For this review, take the finished solid that the model builds, in its own axes (mm). Face numbers are marked on the shaded views. A direction names the side the tool comes from. Give positions to 0.01 mm unless a question says otherwise; leave off trailing zeros. Write each loop counter-clockwise with the first axis right and the second up, starting at its lowest first coordinate (ties: lowest second). Pieces come first, ordered by that corner, then holes.
Q1. Mouldability with a two-part tool opening along Z and no side actions: class the marked faces 1, 2 and 3 as released by +Z, released by -Z, zero draft, split by the parting line, or undercut.
Q2. For line 1 (Z direction, x = 8.5, y = -12); line 2 (Y direction, x = 12.5, z = 1.25); line 3 (Y direction, x = 9.25, z = 7.5), list the stretches that pass through material, from the lowest coordinate up.
Q3. Machinability: for the marked faces 4, 5, 6, 7 and 8, which of the approach directions +Z, -Z, +X, -X, +Y, -Y give a long, thin tool a straight path to every point of the face, cutting with its end or side? Answer none if there is none.
Q4. We need section C-C (x = 13.75). Write out the cut boundary in (y, z).
Q5. We need section A-A (y = -14.25). Write out the cut boundary in (x, z).
Q6. Insertion check: P1, Ø6, axis at x = -6.5, y = -12.5, coming from the +Z side; P2, Ø8, axis at x = -4.5, y = -16.5, coming from the +Z side; P3, Ø1.5, axis at y = -3.5, z = 1.5, coming from the -X side. Each pin has a flat end and moves straight along its axis. Give the tip position at first contact, or say it passes through.
Q7. We need section B-B (x = 1.75). Write out the cut boundary in (y, z).
Q8. We need section D-D (z = 1.75). Write out the cut boundary in (x, y), then the cut area to 3 significant figures.
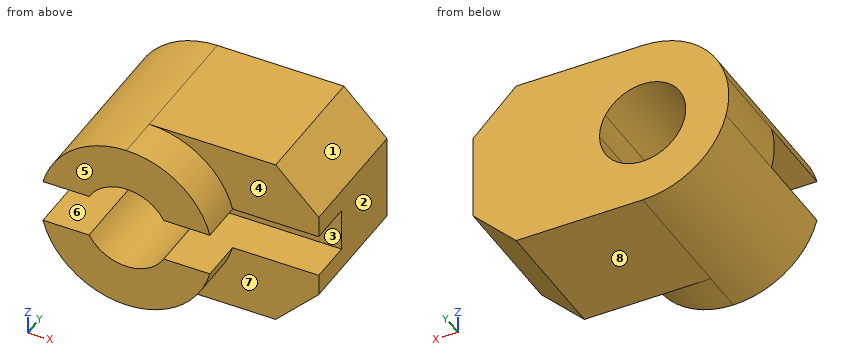
```python
from build123d import *

# Parameters (mm, degrees)
F1_DEPTH = 20
F2_DEPTH = 15
F3_DEPTH = 10


with BuildPart() as f1:
    # F0 (on Front) → F1 (new body)
    with BuildSketch(Plane.XZ):
        with BuildLine():
            ThreePointArc((-4.3301270189, 2.5), (0, 5), (4.3301270189, 2.5))
            Line((4.3301270189, 2.5), (9.6824583655, 2.5))
            ThreePointArc((9.6824583655, 2.5), (6.123724357, 7.9056941504), (0, 10))
            ThreePointArc((0, 10), (-6.123724357, 7.9056941504), (-9.6824583655, 2.5))
            Line((-9.6824583655, 2.5), (-4.3301270189, 2.5))
        make_face()
    extrude(amount=F1_DEPTH)

    # F0 (on Front) → F2 (join)
    with BuildSketch(Plane.XZ):
        with BuildLine():
            ThreePointArc((0, 10), (6.123724357, 7.9056941504), (9.6824583655, 2.5))
            Line((9.6824583655, 2.5), (19.6824583655, 2.5))
            Line((19.6824583655, 2.5), (19.6824583655, 5))
            Line((19.6824583655, 5), (14.6824583655, 10))
            Line((14.6824583655, 10), (0, 10))
        make_face()
    extrude(amount=F2_DEPTH)



with BuildPart() as f1b:
    # F0 (on Front) → F1, piece 2 (new body)
    with BuildSketch(Plane.XZ):
        with BuildLine():
            Line((9.6824583655, -2.5), (4.3301270189, -2.5))
            ThreePointArc((4.3301270189, -2.5), (0, -5), (-4.3301270189, -2.5))
            Line((-4.3301270189, -2.5), (-9.6824583655, -2.5))
            ThreePointArc((-9.6824583655, -2.5), (-6.123724357, -7.9056941504), (0, -10))
            ThreePointArc((0, -10), (6.123724357, -7.9056941504), (9.6824583655, -2.5))
        make_face()
    extrude(amount=F1_DEPTH)

    # F0 (on Front) → F2, piece 2 (join)
    with BuildSketch(Plane.XZ):
        with BuildLine():
            Line((19.6824583655, -2.5), (9.6824583655, -2.5))
            ThreePointArc((9.6824583655, -2.5), (6.123724357, -7.9056941504), (0, -10))
            Line((0, -10), (14.6824583655, -10))
            Line((14.6824583655, -10), (19.6824583655, -5))
            Line((19.6824583655, -5), (19.6824583655, -2.5))
        make_face()
    extrude(amount=F2_DEPTH)


with BuildPart() as f1_1:
    add(f1.part)

    add(f1b.part)  # F3 merges F1b
    # F0 (on Front) → F3 (join)
    with BuildSketch(Plane.XZ):
        with BuildLine():
            ThreePointArc((4.3301270189, 2.5), (4.8296291314, 1.2940952255), (5, 0))
            ThreePointArc((5, 0), (4.8296291314, -1.2940952255), (4.3301270189, -2.5))
            Line((4.3301270189, -2.5), (9.6824583655, -2.5))
            Line((9.6824583655, -2.5), (19.6824583655, -2.5))
            Line((19.6824583655, -2.5), (19.6824583655, 2.5))
            Line((19.6824583655, 2.5), (9.6824583655, 2.5))
            Line((9.6824583655, 2.5), (4.3301270189, 2.5))
        make_face()
        with BuildLine():
            ThreePointArc((-4.3301270189, -2.5), (-5, 0), (-4.3301270189, 2.5))
            Line((-4.3301270189, 2.5), (-9.6824583655, 2.5))
            ThreePointArc((-9.6824583655, 2.5), (-10, 0), (-9.6824583655, -2.5))
            Line((-9.6824583655, -2.5), (-4.3301270189, -2.5))
        make_face()
    extrude(amount=F3_DEPTH)


solid = f1_1.part
```
Computed:
1. face 1: released by +Z
1. face 2: zero draft
1. face 3: undercut
2. line 1: z = -10 to -2.5, 2.5 to 10
2. line 2: y = -10 to 0
2. line 3: y = -15 to 0
3. face 4: +Z, +X, -Y
3. face 5: +Z, -Z, +X, -X, -Y
3. face 6: +X, -X, -Y
3. face 7: -Z, +X, -Y
3. face 8: -Z, +X, -X, +Y, -Y
4. outline: (-15, -10) - (0, -10) - (0, 10) - (-15, 10) - (-15, 2.5) - (-10, 2.5) - (-10, -2.5) - (-15, -2.5) - close
5. outline: (-9.68, -2.5) arc R10 ccw to (0, -10) - (14.68, -10) - (19.68, -5) - (19.68, -2.5) - (4.33, -2.5) arc R5 cw to (-4.33, -2.5) - close; (-9.68, 2.5) - (-4.33, 2.5) arc R5 cw to (4.33, 2.5) - (19.68, 2.5) - (19.68, 5) - (14.68, 10) - (0, 10) arc R10 ccw to start
6. P1: stops at z = 9.37
6. P2: stops at z = 9.99
6. P3: stops at x = -9.97
7. outline: (-20, -9.85) - (-15, -9.85) - (-15, -10) - (0, -10) - (0, -4.68) - (-20, -4.68) - close; (-20, 4.68) - (0, 4.68) - (0, 10) - (-15, 10) - (-15, 9.85) - (-20, 9.85) - close
8. outline: (-9.85, -10) - (-4.68, -10) - (-4.68, 0) - (-9.85, 0) - close; (4.68, -10) - (19.68, -10) - (19.68, 0) - (4.68, 0) - close
8. area: 202 mm2
